Read the model definition and answer for the solid it produces. Units are mm, in the model's axes. A direction names the side the tool comes from. Coordinates: 2 decimals unless noted, no trailing zeros. Write each loop counter-clockwise with the first axis right and the second up, starting at its lowest first coordinate (ties: lowest second). Pieces come first, ordered by that corner, then holes. Notation, with made-up numbers: (19.5, 49) - (48.5, 49) arc R28 ccw to (48.5, 67) - close; hole circle Ø7 at (29, -26.75). An arc over 180 degrees is marked (long way). Return JSON: item names as keys, results as strings.
```python
from build123d import *

# Parameters (mm, degrees)
SKETCH_R      = 1.55
SKETCH_R_2    = 1.5
EXTRUDE_DEPTH = 5
SKETCH001_R   = 5
POCKET_DEPTH  = 2.5
FILLET_R      = 8


with BuildPart() as part:
    # Sketch → Extrude (new body)
    with BuildSketch(Plane.XY):
        with BuildLine():
            ThreePointArc((-8.169873, 2.5), (-17.5, 0), (-8.169873, -2.5))
            Line((8.169873, -2.5), (-8.169873, -2.5))
            ThreePointArc((8.169873, -2.5), (17.5, 0), (8.169873, 2.5))
            Line((-8.169873, 2.5), (8.169873, 2.5))
        make_face()
        with Locations((-12.5, 0)):
            Circle(SKETCH_R, mode=Mode.SUBTRACT)
        with Locations((12.5, 0)):
            Circle(SKETCH_R_2, mode=Mode.SUBTRACT)
    extrude(amount=EXTRUDE_DEPTH)

    # Sketch001 → Pocket (cut)
    with BuildSketch(Plane.XY.offset(5)):
        with Locations((12.5, 0)):
            Circle(SKETCH001_R)
    extrude(amount=-POCKET_DEPTH, mode=Mode.SUBTRACT)

    # Fillet
    fillet_edges = [part.edges().sort_by_distance(p)[0] for p in [
        (-8.169873, 2.5, 2.5),
        (-8.169873, -2.5, 2.5),
        (8.169873, 2.5, 1.25),
        (8.169873, -2.5, 1.25),
    ]]
    fillet(fillet_edges, radius=FILLET_R)


solid = part.part
```
(1) Straight lines are drawn through the part: line 1 (Y direction, x = -12.5, z = 3.6); line 2 (X direction, y = 0.25, z = 1.7); line 3 (Z direction, x = 15, y = 2.5). For each, find the intervals that lie inside material, in ascending order. Write a range as from..to.
Answer:
{"line 1": "-5..-1.55, 1.55..5", "line 2": "-17.49..-14.03, -10.97..11.02, 13.98..17.49", "line 3": "0..2.5"}
(2) A cutting plane is placed at C-C (y = 0). Determine the outline of the cut face in (x, z).
Answer:
{"outline": "(-17.5, 0) - (-14.05, 0) - (-14.05, 5) - (-17.5, 5) - close; (-10.95, 0) - (11, 0) - (11, 2.5) - (7.5, 2.5) - (7.5, 5) - (-10.95, 5) - close; (14, 0) - (17.5, 0) - (17.5, 2.5) - (14, 2.5) - close"}
(3) A cutting plane is placed at D-D (z = 2.95). Determine the outline of the cut face in (x, y), and give its area (3 significant figures).
Answer:
{"outline": "(-9.55, -4.04) arc R8 cw to (-4.84, -2.5) - (8.17, -2.5) arc R5 cw to (8.17, 2.5) - (-4.84, 2.5) arc R8 cw to (-9.55, 4.04) arc R5 ccw (long way) to start; hole circle Ø3.1 at (-12.5, 0)", "area": "150 mm²"}
(4) Flat-ended cylindrical pins translate along their axes: P1, Ø2.5, axis at x = 12.5, y = 0, coming from the -Z side; P2, Ø2, axis at y = -3, z = 2, coming from the -X side; P3, Ø1.5, axis at x = -6.5, z = 1.5, coming from the +Y side; P4, Ø1.5, axis at x = -1, z = 2, coming from the -Y side. Find the tip coordinate at first contact, or state that the pin passes through.
Answer:
{"P1": "through", "P2": "x = -17.08", "P3": "y = 2.87", "P4": "y = -2.5"}
(5) Determine the mould class of faces 1 (the face through (0, 0, 0)), 2 (the face through (7.5, 0, 3.8)), 3 (the face through (7.349, 2.905, 1.268)) for opening direction X: +X half, -X half, draft (parallel to the pull), parting line (faces both ways), or undercut.
Answer:
{"face 1": "draft", "face 2": "+X half", "face 3": "undercut"}
(6) A cutting plane is placed at B-B (z = 1.65). Determine the outline of the cut face in (x, y), and give its area (3 significant figures).
Answer:
{"outline": "(-9.55, -4.04) arc R8 cw to (-4.84, -2.5) - (4.84, -2.5) arc R8 cw to (9.55, -4.04) arc R5 ccw (long way) to (9.55, 4.04) arc R8 cw to (4.84, 2.5) - (-4.84, 2.5) arc R8 cw to (-9.55, 4.04) arc R5 ccw (long way) to start; hole circle Ø3.1 at (-12.5, 0); hole circle Ø3 at (12.5, 0)", "area": "224 mm²"}
(7) Which of the six approach directions +Z, -Z, +X, -X, +Y, -Y give full straight-line access (tool end or side, diameter ignored) to faces 4 (the face through (-7.349, 2.905, 2.535)), 5 (the face through (-17.498, 0.154, 2.465)), 6 (the face through (7.349, -2.905, 1.268))?
Answer:
{"face 4": "+Z, -Z, +Y", "face 5": "+Z, -Z", "face 6": "+Z, -Z, -Y"}
(8) A cutting plane is placed at A-A (x = -12.5). Determine the outline of the cut face in (y, z), and give its area (3 significant figures).
Answer:
{"outline": "(-5, 0) - (-1.55, 0) - (-1.55, 5) - (-5, 5) - close; (1.55, 0) - (5, 0) - (5, 5) - (1.55, 5) - close", "area": "34.5 mm²"}
